from build123d import *

# Parameters (mm, degrees)
BOSS_EXTRUDE1_DEPTH = 38.1
CUT_EXTRUDE1_REACH  = 5.175
SKETCH3_R           = 4.365625


with BuildPart() as part:
    # Sketch1 → Boss-Extrude1 (new body, symmetric)
    with BuildSketch(Plane(origin=(0, 0, 0), x_dir=(-1, 0, 0), z_dir=(0, 0, 1))):
        Polygon((0, 0), (-38.1, 0), (-38.1, -3.175), (-3.175, -3.175), (-3.175, -38.1), (0, -38.1), align=None)
    extrude(amount=BOSS_EXTRUDE1_DEPTH, both=True)

    # Sketch3 → Cut-Extrude1 (cut, up to next)
    with BuildSketch(Plane(origin=(0, 3.175, 0), x_dir=(1, 0, 0), z_dir=(0, 1, 0)), mode=Mode.PRIVATE) as cut_extrude1_sk1:
        with Locations(Location((25.4, 0, 0), (0, 0, 270))):  # turned: the seam where the file's is
            Circle(SKETCH3_R)
    cut_extrude1_tool1 = extrude(cut_extrude1_sk1.sketch, amount=-CUT_EXTRUDE1_REACH, mode=Mode.PRIVATE) & part.part
    add(cut_extrude1_tool1.solids().sort_by_distance((25.4, 3.175, 0))[0], mode=Mode.SUBTRACT)


solid = part.part
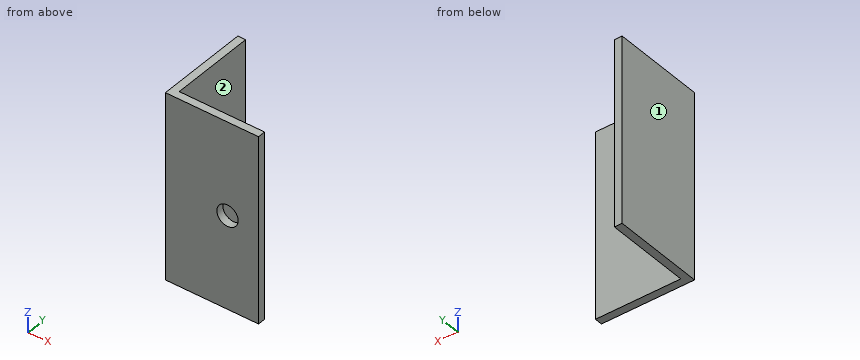
Work out the finished part from the listing and answer in its coordinate system (mm). Face numbers are marked on the shaded views. A direction names the side the tool comes from. Round coordinates to 2 decimals unless told otherwise and drop trailing zeros. Write each loop counter-clockwise with the first axis right and the second up, starting at its lowest first coordinate (ties: lowest second). Pieces come first, ordered by that corner, then holes. Notation, with made-up numbers: (69, -24.75) -> (81, -24.75) arc R8 cw to (81, -10.75) -> close; hole circle Ø5 at (66.5, 34). An arc over 180 degrees is marked (long way). Answer as CSV lines item,"result". Start each with the question number.
(1) Find the intervals of material crossed by probe 1 along X at (y, z) = (2, 0); probe 2 along Y at (x, z) = (5, -0.5) (3 decimals), in increasing order.
(2) The part is cut by section D-D, the plane y = 29. Give the vertices of the cut face in (x, z) (3 decimals).
(3) The part is cut by section C-C, the plane z = 27. Give the vertices of the cut face in (x, y) (3 decimals).
(4) Each of these flat-tipped pins is pushed along its axis until it touches: pin 1 (10.5 mm diameter, centred on y = 23, z = -5, fed in from +X) (3 decimals); pin 2 (10 mm diameter, centred on x = 25.4, z = 0, fed in from +Y) (3 decimals). Where does it stop, or does it pass through?
(5) The part is cut by section B-B, the plane z = 0. Give the vertices of the cut face in (x, y) (3 decimals).
(6) The part is cut by section A-A, the plane x = 25.4. Give the vertices of the cut face in (y, z) (3 decimals), then the cut area to 3 significant figures.
(7) A tool of negligible diameter and unlimited length cuts with its end or side. For the marked faces 1 and 2, from which of +Z, -Z, +X, -X, +Y, -Y can it reach the whole face along a straight path? Write none if from no direction.
Output values:
1,probe 1,"x = 0 to 21.03, 29.77 to 38.1"
1,probe 2,"y = 0 to 3.175"
2,outline,"(0, -38.1) -> (3.175, -38.1) -> (3.175, 38.1) -> (0, 38.1) -> close"
3,outline,"(0, 0) -> (38.1, 0) -> (38.1, 3.175) -> (3.175, 3.175) -> (3.175, 38.1) -> (0, 38.1) -> close"
4,pin 1,"stops at x = 3.175"
4,pin 2,"stops at y = 3.175"
5,outline,"(0, 0) -> (21.034, 0) -> (21.034, 3.175) -> (3.175, 3.175) -> (3.175, 38.1) -> (0, 38.1) -> close; (29.766, 0) -> (38.1, 0) -> (38.1, 3.175) -> (29.766, 3.175) -> close"
6,outline,"(0, -38.1) -> (3.175, -38.1) -> (3.175, -4.366) -> (0, -4.366) -> close; (0, 4.366) -> (3.175, 4.366) -> (3.175, 38.1) -> (0, 38.1) -> close"
6,area,"214 mm²"
7,face 1,"+Z, -Z, -X, +Y, -Y"
7,face 2,"+Z, -Z, +X, +Y"
